Here's how the part is built. I have some questions about the finished solid (model axes, mm). Coordinates: 2 decimals unless noted, no trailing zeros. Write each loop counter-clockwise with the first axis right and the second up, starting at its lowest first coordinate (ties: lowest second). Pieces come first, ordered by that corner, then holes.
Item 1: If we section it at B-B (y = 4.25): Count the separate pieces of the cut face and the enclosed holes in it, then the cut area to 3 significant figures.
Item 2: If I drill on line 1 (Z direction, x = -130, y = -0.95); line 2 (Z direction, x = -38, y = 3.25); line 3 (Y direction, x = -3, z = 0), over which ranges is the centre line in solid material (lowest first)?
Item 3: If we section it at A-A (x = -120): Please give me the cut outline in (y, z).
Item 4: I'm going to push flat-ended pins straight in: pin 1 Ø1.1 at (x, y) = (1, 4) entering from -Z; pin 2 Ø3.5 at (x, z) = (-130, -1.5) entering from +Y; pin 3 Ø4.5 at (x, z) = (0, 0) entering from -Y. Where does each tip first touch, or does it pass through?
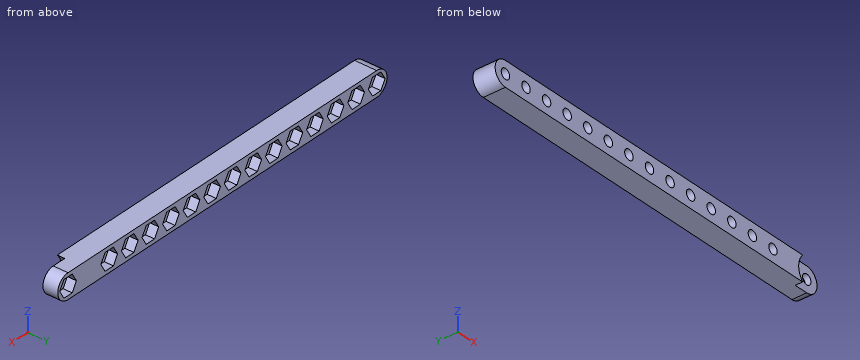
from build123d import *

# Parameters (mm, degrees)
SKETCH1_R           = 2.05
BOSS_EXTRUDE1_DEPTH = 6
CUT_EXTRUDE1_DEPTH  = 3.7
BOSS_EXTRUDE2_START = 3
BOSS_EXTRUDE2_DEPTH = 3
SKETCH5_R           = 2.05
CUT_EXTRUDE2_DEPTH  = 156.341559153


with BuildPart() as part:
    # Sketch1 → Boss-Extrude1 (new body)
    with BuildSketch(Plane(origin=(0, 0, 0), x_dir=(1, 0, 0), z_dir=(0, 1, 0))):
        with BuildLine():
            Line((0, -5), (-150, -5))
            ThreePointArc((-150, -5), (-155, 0), (-150, 5))
            Line((-150, 5), (0, 5))
            ThreePointArc((0, 5), (5, 0), (0, -5))
        make_face()
        with Locations(Location((0, 0, 0), (0, 0, 270))):
            Circle(SKETCH1_R, mode=Mode.SUBTRACT)
        with Locations(Location((-50, 0, 0), (0, 0, 270))):
            Circle(SKETCH1_R, mode=Mode.SUBTRACT)
        with Locations(Location((-60, 0, 0), (0, 0, 270))):
            Circle(SKETCH1_R, mode=Mode.SUBTRACT)
        with Locations(Location((-70, 0, 0), (0, 0, 270))):
            Circle(SKETCH1_R, mode=Mode.SUBTRACT)
        with Locations(Location((-80, 0, 0), (0, 0, 270))):
            Circle(SKETCH1_R, mode=Mode.SUBTRACT)
        with Locations(Location((-90, 0, 0), (0, 0, 270))):
            Circle(SKETCH1_R, mode=Mode.SUBTRACT)
        with Locations(Location((-100, 0, 0), (0, 0, 270))):
            Circle(SKETCH1_R, mode=Mode.SUBTRACT)
        with Locations(Location((-110, 0, 0), (0, 0, 270))):
            Circle(SKETCH1_R, mode=Mode.SUBTRACT)
        with Locations(Location((-120, 0, 0), (0, 0, 270))):
            Circle(SKETCH1_R, mode=Mode.SUBTRACT)
        with Locations(Location((-130, 0, 0), (0, 0, 270))):
            Circle(SKETCH1_R, mode=Mode.SUBTRACT)
        with Locations(Location((-140, 0, 0), (0, 0, 270))):
            Circle(SKETCH1_R, mode=Mode.SUBTRACT)
        with Locations(Location((-150, 0, 0), (0, 0, 270))):
            Circle(SKETCH1_R, mode=Mode.SUBTRACT)
        with Locations(Location((-20, 0, 0), (0, 0, 270))):
            Circle(SKETCH1_R, mode=Mode.SUBTRACT)
        with Locations(Location((-30, 0, 0), (0, 0, 270))):
            Circle(SKETCH1_R, mode=Mode.SUBTRACT)
        with Locations(Location((-40, 0, 0), (0, 0, 270))):
            Circle(SKETCH1_R, mode=Mode.SUBTRACT)
    extrude(amount=BOSS_EXTRUDE1_DEPTH)

    # Sketch2 → Cut-Extrude1 (cut)
    with BuildSketch(Plane(origin=(0, 6, 0), x_dir=(1, 0, 0), z_dir=(0, 1, 0))):
        Polygon((4.041451884, 0), (2.020725942, 3.5), (-2.020725942, 3.5), (-4.041451884, 0), (-2.020725942, -3.5), (2.020725942, -3.5), align=None)
        Polygon((-45.958548116, 0), (-47.979274058, 3.5), (-52.020725942, 3.5), (-54.041451884, 0), (-52.020725942, -3.5), (-47.979274058, -3.5), align=None)
        Polygon((-55.958548116, 0), (-57.979274058, 3.5), (-62.020725942, 3.5), (-64.041451884, 0), (-62.020725942, -3.5), (-57.979274058, -3.5), align=None)
        Polygon((-65.958548116, 0), (-67.979274058, 3.5), (-72.020725942, 3.5), (-74.041451884, 0), (-72.020725942, -3.5), (-67.979274058, -3.5), align=None)
        Polygon((-75.958548116, 0), (-77.979274058, 3.5), (-82.020725942, 3.5), (-84.041451884, 0), (-82.020725942, -3.5), (-77.979274058, -3.5), align=None)
        Polygon((-85.958548116, 0), (-87.979274058, 3.5), (-92.020725942, 3.5), (-94.041451884, 0), (-92.020725942, -3.5), (-87.979274058, -3.5), align=None)
        Polygon((-95.958548116, 0), (-97.979274058, 3.5), (-102.020725942, 3.5), (-104.041451884, 0), (-102.020725942, -3.5), (-97.979274058, -3.5), align=None)
        Polygon((-105.958548116, 0), (-107.979274058, 3.5), (-112.020725942, 3.5), (-114.041451884, 0), (-112.020725942, -3.5), (-107.979274058, -3.5), align=None)
        Polygon((-115.958548116, 0), (-117.979274058, 3.5), (-122.020725942, 3.5), (-124.041451884, 0), (-122.020725942, -3.5), (-117.979274058, -3.5), align=None)
        Polygon((-125.958548116, 0), (-127.979274058, 3.5), (-132.020725942, 3.5), (-134.041451884, 0), (-132.020725942, -3.5), (-127.979274058, -3.5), align=None)
        Polygon((-135.958548116, 0), (-137.979274058, 3.5), (-142.020725942, 3.5), (-144.041451884, 0), (-142.020725942, -3.5), (-137.979274058, -3.5), align=None)
        Polygon((-145.958548116, 0), (-147.979274058, 3.5), (-152.020725942, 3.5), (-154.041451884, 0), (-152.020725942, -3.5), (-147.979274058, -3.5), align=None)
        Polygon((-15.958548116, 0), (-17.979274058, 3.5), (-22.020725942, 3.5), (-24.041451884, 0), (-22.020725942, -3.5), (-17.979274058, -3.5), align=None)
        Polygon((-25.958548116, 0), (-27.979274058, 3.5), (-32.020725942, 3.5), (-34.041451884, 0), (-32.020725942, -3.5), (-27.979274058, -3.5), align=None)
        Polygon((-35.958548116, 0), (-37.979274058, 3.5), (-42.020725942, 3.5), (-44.041451884, 0), (-42.020725942, -3.5), (-37.979274058, -3.5), align=None)
    extrude(amount=-CUT_EXTRUDE1_DEPTH, mode=Mode.SUBTRACT)

    # Sketch4 → Boss-Extrude2 (add)
    with BuildSketch(Plane.XZ.offset(BOSS_EXTRUDE2_START)):
        with BuildLine():
            Line((-150, 5), (-5.577689938, 5))
            ThreePointArc((-5.577689938, 5), (-7.490702573, 0), (-5.577689938, -5))
            Line((-5.577689938, -5), (-150, -5))
            ThreePointArc((-150, -5), (-155, 0), (-150, 5))
        make_face()
    extrude(amount=-BOSS_EXTRUDE2_DEPTH)

    # Sketch5 → Cut-Extrude2 (cut, through all)
    with BuildSketch(Plane.XZ.offset(3)):
        with Locations(Location((-50, 0, 0), (0, 0, 270))):
            Circle(SKETCH5_R)
        with Locations(Location((-60, 0, 0), (0, 0, 270))):
            Circle(SKETCH5_R)
        with Locations(Location((-70, 0, 0), (0, 0, 270))):
            Circle(SKETCH5_R)
        with Locations(Location((-80, 0, 0), (0, 0, 270))):
            Circle(SKETCH5_R)
        with Locations(Location((-90, 0, 0), (0, 0, 270))):
            Circle(SKETCH5_R)
        with Locations(Location((-100, 0, 0), (0, 0, 270))):
            Circle(SKETCH5_R)
        with Locations(Location((-110, 0, 0), (0, 0, 270))):
            Circle(SKETCH5_R)
        with Locations(Location((-120, 0, 0), (0, 0, 270))):
            Circle(SKETCH5_R)
        with Locations(Location((-130, 0, 0), (0, 0, 270))):
            Circle(SKETCH5_R)
        with Locations(Location((-140, 0, 0), (0, 0, 270))):
            Circle(SKETCH5_R)
        with Locations(Location((-150, 0, 0), (0, 0, 270))):
            Circle(SKETCH5_R)
        with Locations(Location((-40, 0, 0), (0, 0, 270))):
            Circle(SKETCH5_R)
        with Locations(Location((-30, 0, 0), (0, 0, 270))):
            Circle(SKETCH5_R)
        with Locations(Location((-20, 0, 0), (0, 0, 270))):
            Circle(SKETCH5_R)
    extrude(amount=-CUT_EXTRUDE2_DEPTH, mode=Mode.SUBTRACT)


solid = part.part
Answer list:
1. separate pieces: 1
1. enclosed holes: 15
1. area: 942 mm2
2. line 1: z = -5 to -2.05, 2.05 to 5
2. line 2: z = -5 to -3.5, 3.5 to 5
2. line 3: y = 0 to 2.3
3. outline: (-3, -5) - (6, -5) - (6, -3.5) - (2.3, -3.5) - (2.3, -2.05) - (-3, -2.05) - close; (-3, 2.05) - (2.3, 2.05) - (2.3, 3.5) - (6, 3.5) - (6, 5) - (-3, 5) - close
4. pin 1: stops at z = -4.98
4. pin 2: stops at y = 2.3
4. pin 3: stops at y = 0
